```python
from build123d import *

# Parameters (mm, degrees)
F1_DEPTH = 63.5
F2_DEPTH = 25.4
F3_DEPTH = 44.45
F0_W     = 27.7197288275
F0_H     = 28.575
F5_R     = 6.35


with BuildPart() as f1:
    # F0 (on Front) → F1 (new body, symmetric)
    with BuildSketch(Plane.XZ):
        Polygon((-41.275, -9.525), (41.275, -9.525), (41.275, 9.525), (22.225, 9.525), (-41.275, 9.525), align=None)
    extrude(amount=F1_DEPTH, both=True)

    # F0 (on Front) → F2 (join, symmetric)
    with BuildSketch(Plane.XZ):
        with BuildLine():
            add(Edge.make_bspline(
                [(-41.275, 9.525), (-8.7416619248, 26.8411315561), (18.6592967194, 61.1014551348), (56.1959573796, 61.8994668263)],
                knots=[0, 0, 0, 0, 110.5640017612, 110.5640017612, 110.5640017612, 110.5640017612], degree=3))
            Line((-41.275, 9.525), (22.225, 9.525))
            Line((22.225, 9.525), (22.225, 26.9875))
            ThreePointArc((22.225, 26.9875), (32.1192632598, 51.3435637879), (56.1959573796, 61.8994668263))
        make_face()
    extrude(amount=F2_DEPTH, both=True)

    # F0 (on Front) → F3 (join, symmetric)
    with BuildSketch(Plane.XZ):
        with BuildLine():
            Line((22.225, 9.525), (41.275, 9.525))
            Line((41.275, 9.525), (41.275, 26.9875))
            ThreePointArc((41.275, 26.9875), (45.9246798487, 38.2128201513), (57.15, 42.8625))
            Line((57.15, 42.8625), (60.325, 42.8625))
            Line((60.325, 42.8625), (60.325, 61.9125))
            Line((60.325, 61.9125), (57.15, 61.9125))
            add(Edge.make_bspline(
                [(56.1959573796, 61.8994668263), (56.513244332, 61.9062121971), (56.8312554651, 61.9105667358), (57.15, 61.9125)],
                knots=[110.5640017612, 110.5640017612, 110.5640017612, 110.5640017612, 111.4985685166, 111.4985685166, 111.4985685166, 111.4985685166], degree=3))
            ThreePointArc((56.1959573796, 61.8994668263), (32.1192632598, 51.3435637879), (22.225, 26.9875))
            Line((22.225, 26.9875), (22.225, 9.525))
        make_face()
    extrude(amount=F3_DEPTH, both=True)

    # F0 (on Front) → F4 (revolve)
    with BuildSketch(Plane.XZ):
        with Locations((97.2651355863, 52.3875)):
            Rectangle(F0_W, F0_H)
    revolve(axis=Axis((83.4052711725, 0, 52.3875), (0, 0, 1)))

    # F5
    f5_edges = [f1.edges().sort_by_distance(p)[0] for p in [
        (41.275, -63.5, 0),
        (-41.275, -63.5, 0),
        (-41.275, 63.5, 0),
        (41.275, 63.5, 0),
    ]]
    fillet(f5_edges, radius=F5_R)


solid = f1.part
```
Verification items for the finished model (mm, model axes). A direction names the side the tool comes from. Coordinates: 2 decimals unless noted, no trailing zeros. Loops run counter-clockwise (first coordinate to the right, second up) from the corner with the lowest first, then second, coordinate; pieces in that order, holes last. Notation, with made-up numbers: (16.25, 28.5) -> (67.25, 28.5) arc R13 cw to (67.25, 33.5) -> close; hole circle Ø8 at (-29.75, -3.5). An arc over 180 degrees is marked (long way). Answer in a Markdown table with one row per item. Add a question column.
1. Section check B-B, the plane x = 88.5. Enter the section's corners in (y, z) (3 decimals), then the cut area to 3 significant figures.
2. Material ranges on probe 1 along Y at (x, z) = (11, 10); probe 2 along X at (y, z) = (-35, -3) (3 decimals); probe 3 along Z at (x, y) = (-21, -30.5) (3 decimals), recorded low to high. Write a range as [from, to].
3. Draft check along X on faces 1 (the face through (1, 44, 9.525)), 2 (the face through (45.802, -0.622, 38.089)), 3 (the face through (-39.464, -61.59, -0.133)), 4 (the face through (39.464, -61.59, 0.133)). Enter one of: +X half, -X half, draft (parallel to the pull), parting line (faces both ways), or undercut.
4. Section check A-A, the plane z = 7. Enter the section's corners in (x, y) (3 decimals), then the cut area to 3 significant figures.
5. Depth check by flat-ended pin: P1, Ø19, axis at x = 38.5, z = 36, coming from the -Y side; P2, Ø1, axis at x = 67.5, z = 39.5, coming from the +Y side; P3, Ø1, axis at x = 58.5, y = 18.5, coming from the +Z side. Enter the tip coordinate at first touch or a pass-through.
6. Access from +Z, -Z, +X, -X, +Y, -Y to the whole of each face (thin tool, end or side, straight path). Record for faces 5 (the face through (22.225, 35, 18)), 6 (the face through (22.225, -35, 18)), 7 (the face through (37, 44.45, 36)).
Derived:
| question | item | result |
|---|---|---|
| 1 | outline | (-27.248, 38.1) -> (27.248, 38.1) -> (27.248, 66.675) -> (-27.248, 66.675) -> close |
| 1 | area | 1,560 mm² |
| 2 | probe 1 | y = [-25.4, 25.4] |
| 2 | probe 2 | x = [-41.275, 41.275] |
| 2 | probe 3 | z = [-9.525, 9.525] |
| 3 | face 1 | draft |
| 3 | face 2 | undercut |
| 3 | face 3 | -X half |
| 3 | face 4 | +X half |
| 4 | outline | (-41.275, -57.15) arc R6.35 ccw to (-34.925, -63.5) -> (34.925, -63.5) arc R6.35 ccw to (41.275, -57.15) -> (41.275, 57.15) arc R6.35 ccw to (34.925, 63.5) -> (-34.925, 63.5) arc R6.35 ccw to (-41.275, 57.15) -> close |
| 4 | area | 10,400 mm² |
| 5 | P1 | stops at y = -44.45 |
| 5 | P2 | stops at y = 23.04 |
| 5 | P3 | stops at z = 61.91 |
| 6 | face 5 | +Z, -X, +Y |
| 6 | face 6 | +Z, -X, -Y |
| 6 | face 7 | +Z, +X, -X, +Y |
